```python
from build123d import *

# Parameters (mm, degrees)
F0_W     = 68
F0_H     = 53
F1_DEPTH = 1.5875
F2_DEPTH = 26


# Not quite as in the source:
# - a length typed as a fraction of an inch, garbled in the dataset ("3 / 203.2 mm" for 3/8 in), is restored


with BuildPart() as f1:
    # F0 (on Top) → F1 (new body)
    with BuildSketch(Plane.XY):
        Polygon((0, 150), (0, 0), (38.399413228, 0), (38.399413228, 53), (106.399413228, 53), (106.399413228, 0), (140, 0), (140, 150), align=None)
        with Locations((72.399413228, 26.5)):
            Rectangle(F0_W, F0_H)
    extrude(amount=F1_DEPTH)

    # F0 (on Top) → F2 (join)
    with BuildSketch(Plane.XY):
        with Locations((72.399413228, 26.5)):
            Rectangle(F0_W, F0_H)
    extrude(amount=F2_DEPTH)


solid = f1.part
```
The listing builds one solid part. Answer for the finished solid, in the listing's coordinates (mm). A direction names the side the tool comes from. Coordinates: 2 decimals unless noted, no trailing zeros. Order: outer loops, then holes, each group sorted by start corner. A loop starts at its lowest first (then second) coordinate and runs counter-clockwise, first axis right, second up. Notation, with made-up numbers: M 47,-28 L 76,-28 A18 ccw 76,-11 Z; hole C 86,32 d3. An arc over 180 degrees is marked long. Answer as a JSON object with one key per item and string values. Group by question number.
1. Straight lines are drawn through the part: line 1 (Z direction, x = 13.5, y = 7.5); line 2 (Y direction, x = 70, z = 16.5); line 3 (X direction, y = 7, z = 23.5). For each, find the intervals that lie inside material, in ascending order.
2. A tool of negligible diameter and unlimited length cuts with its end or side. For faces 1 (the flat face through (72, 53, 14)), 2 (the flat face through (69, 0, 13)), 3 (the flat face through (106.399, 26, 14)), 4 (the flat face through (38.399, 26, 14)), from which of +Z, -Z, +X, -X, +Y, -Y can it reach the whole face along a straight path? Write none if from no direction.
3. Section A-A on y = 24.5 is taken. Write down the section's boundary in (x, z), then the cut area to 3 significant figures.
4. Section D-D on y = 117 is taken. Write down the section's boundary in (x, z), then the cut area to 3 significant figures.
5. Section C-C on x = 53.5 is taken. Write down the section's boundary in (y, z).
6. Section B-B on z = 20.5 is taken. Write down the section's boundary in (x, y).
7. Flat-ended cylindrical pins translate along their axes: P1, Ø12, axis at y = 14.5, z = 16, coming from the +X side; P2, Ø1.5, axis at x = 112.5, y = 22.5, coming from the +Z side; P3, Ø12, axis at x = 29, z = 21.5, coming from the +Y side; P4, Ø7.5, axis at x = 66.5, z = 11.5, coming from the +Y side. Find the tip coordinate at first contact, or state that the pin passes through.
Values follow:
{
 "1": {"line 1": "0 to 1.59", "line 2": "0 to 53", "line 3": "38.4 to 106.4"},
 "2": {"face 1": "+Z, +X, -X, +Y", "face 2": "+Z, -Z, +X, -X, -Y", "face 3": "+Z, +X, +Y, -Y", "face 4": "+Z, -X, +Y, -Y"},
 "3": {"outline": "M 0,0 L 140,0 L 140,1.59 L 106.4,1.59 L 106.4,26 L 38.4,26 L 38.4,1.59 L 0,1.59 Z", "area": "1,880 mm2"},
 "4": {"outline": "M 0,0 L 140,0 L 140,1.59 L 0,1.59 Z", "area": "222 mm2"},
 "5": {"outline": "M 0,0 L 150,0 L 150,1.59 L 53,1.59 L 53,26 L 0,26 Z"},
 "6": {"outline": "M 38.4,0 L 106.4,0 L 106.4,53 L 38.4,53 Z"},
 "7": {"P1": "x = 106.4", "P2": "z = 1.59", "P3": "through", "P4": "y = 53"}
}
